Input: part model. Units: mm. Frame: model coordinates. Face numbers are marked on the shaded views. A direction names the side the tool comes from. Round coordinates to 2 decimals unless told otherwise and drop trailing zeros. Loops run counter-clockwise (first coordinate to the right, second up) from the corner with the lowest first, then second, coordinate; pieces in that order, holes last. Notation, with made-up numbers: M 1.5,34.5 L 46.5,34.5 A5 ccw 46.5,42.5 Z; hole C -5,35.5 d7. An arc over 180 degrees is marked long. Use one line per item in the form item = value. Start each with the question number.
Q1. Access query for the marked faces 1 and 2. Directions: +Z, -Z, +X, -X, +Y, -Y. A direction counts if a zero-diameter tool reaches every point of the face in a straight line with its end or side. Return the directions, or none.
Q2. Section query A-A, the plane x = 67.25. Output: boundary loops of the cut face in (y, z), and give its area (3 significant figures).
Q3. Section query B-B, the plane z = -7.75. Output: boundary loops of the cut face in (x, y).
Q4. Ray query, line 1 along Z through (x, y) = (-2, 0); line 2 along Y through (x, z) = (60, -2.15); line 3 along Z through (x, y) = (20, -2). Return the intervals inside material, ascending.
Q5. First-contact query: P1, Ø2, axis at y = -2, z = -15.5, coming from the -X side; P2, Ø10, axis at y = -16.5, z = -7, coming from the +X side; P3, Ø10, axis at x = -7, z = -10.5, coming from the +Y side; P4, Ø18, axis at x = -4.5, y = -9, coming from the -Z side. Flat tips, straight axial feed; report the tip coordinate or a pass-through.
Q6. Mould query, pull axis Z, two halves, no side actions, for the marked faces 3, 4, 5 and 6. Classes: pulls with the +Z half, pulls with the -Z half, needs draft (parallel to the pull), parting line crosses it, or undercut.
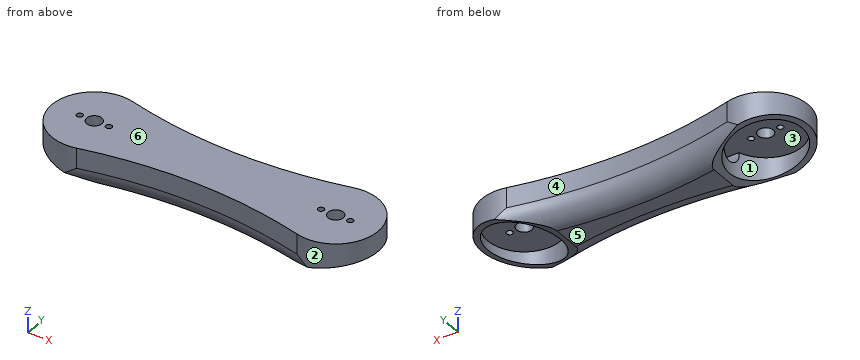
```python
from build123d import *

# Parameters (mm, degrees)
SALIENTE_EXTRUIR1_DEPTH    = 20
CORTAR_EXTRUIR1_DEPTH      = 87.034876649
CORTAR_EXTRUIR1_DEPTH_BACK = 87.034876649
CROQUIS4_R                 = 18
CORTAR_EXTRUIR2_DEPTH      = 14
CROQUIS5_R                 = 3.75
CROQUIS5_R_2               = 1.5
CORTAR_EXTRUIR3_DEPTH      = 85.841027952
REDONDEO1_R                = 10
CORTAR_EXTRUIR4_DEPTH      = 47


with BuildPart() as part:
    # Croquis1 → Saliente-Extruir1 (new body)
    with BuildSketch(Plane.XY):
        with BuildLine():
            ThreePointArc((54.87804878, 20.365795239), (0, 13.570744225), (-54.87804878, 20.365795239))
            ThreePointArc((-54.87804878, 20.365795239), (-81, 0), (-54.87804878, -20.365795239))
            ThreePointArc((-54.87804878, -20.365795239), (0, -13.570744225), (54.87804878, -20.365795239))
            ThreePointArc((54.87804878, -20.365795239), (81, 0), (54.87804878, 20.365795239))
        make_face()
    extrude(amount=-SALIENTE_EXTRUIR1_DEPTH)

    # Croquis2 → Cortar-Extruir1 (cut, two sides: drawn at the far end of the back side and taken through both)
    with BuildSketch(Plane(origin=(0, 0, 0), x_dir=(1, 0, 0), z_dir=(0, 1, 0)).offset(-CORTAR_EXTRUIR1_DEPTH_BACK)):
        with BuildLine():
            Line((-81, 10), (-81, 20))
            Line((-81, 20), (-39, 20))
            ThreePointArc((-39, 20), (-59.790503904, 14.120116398), (-81, 10))
        make_face()
        with BuildLine():
            Line((81, 10), (81, 20))
            Line((81, 20), (39, 20))
            ThreePointArc((39, 20), (59.790503904, 14.120116398), (81, 10))
        make_face()
    extrude(amount=CORTAR_EXTRUIR1_DEPTH + CORTAR_EXTRUIR1_DEPTH_BACK, mode=Mode.SUBTRACT)

    # Croquis4 → Cortar-Extruir2 (cut)
    with BuildSketch(Plane(origin=(0, 0, -20), x_dir=(-1, 0, 0), z_dir=(0, 0, -1))):
        with Locations((60, 0)):
            Circle(CROQUIS4_R)
        with Locations((-60, 0)):
            Circle(CROQUIS4_R)
    extrude(amount=-CORTAR_EXTRUIR2_DEPTH, mode=Mode.SUBTRACT)

    # Croquis5 → Cortar-Extruir3 (cut, through all)
    with BuildSketch(Plane(origin=(0, 0, -6), x_dir=(-1, 0, 0), z_dir=(0, 0, -1))):
        with Locations((60, 0)):
            Circle(CROQUIS5_R)
        with Locations((67.25, 0)):
            Circle(CROQUIS5_R_2)
        with Locations(Location((52.75, 0, 0), (0, 0, 180))):
            Circle(CROQUIS5_R_2)
        with Locations(Location((-67.25, 0, 0), (0, 0, 180))):
            Circle(CROQUIS5_R_2)
        with Locations(Location((-60, 0, 0), (0, 0, 180))):
            Circle(CROQUIS5_R)
        with Locations((-52.75, 0)):
            Circle(CROQUIS5_R_2)
    extrude(amount=-CORTAR_EXTRUIR3_DEPTH, mode=Mode.SUBTRACT)

    # Redondeo1
    # the kernel refuses this fillet: 10 mm, written as the material it takes off along each edge
    with BuildSketch(Plane(origin=(0, -238.570744225, -20), x_dir=(-0.28147080374244887, 0.9595697924802447, 0), z_dir=(-0.9595697924802447, -0.28147080374244887, 0))) as redondeo1_piece_1:
        with BuildLine():
            CenterArc((225 + REDONDEO1_R, -REDONDEO1_R), REDONDEO1_R, 90, 90)
            Line((225, -REDONDEO1_R), (225, 0))
            Line((225, 0), (225 + REDONDEO1_R, 0))
        make_face()
    revolve(axis=Axis((0, -238.570744225, -20), (0, 0, -1)), revolution_arc=32.696012994, mode=Mode.SUBTRACT)
    with BuildSketch(Plane(origin=(0, 238.570744225, -20), x_dir=(0.28147080374244876, -0.9595697924802447, 0), z_dir=(0.9595697924802447, 0.28147080374244876, 0))) as redondeo1_piece_2:
        with BuildLine():
            CenterArc((225 + REDONDEO1_R, -REDONDEO1_R), REDONDEO1_R, 90, 90)
            Line((225 + REDONDEO1_R, 0), (225, 0))
            Line((225, 0), (225, -REDONDEO1_R))
        make_face()
    revolve(axis=Axis((0, 238.570744225, -20), (0, 0, -1)), revolution_arc=32.696012994, mode=Mode.SUBTRACT)

    # Croquis6 → Cortar-Extruir4 (cut, symmetric)
    with BuildSketch(Plane(origin=(0, 0, 0), x_dir=(0, 0, -1), z_dir=(1, 0, 0))):
        with BuildLine():
            Line((6, 5.5), (6, -5.5))
            ThreePointArc((6, -5.5), (13, 0), (6, 5.5))
        make_face()
    extrude(amount=CORTAR_EXTRUIR4_DEPTH, both=True, mode=Mode.SUBTRACT)


solid = part.part
```
Results found:
q1.face_1 = -Z
q1.face_2 = +Z, -Z
q2.outline = M -19.71,-12.46 L -16.48,-12.46 L -16.48,-6 L -1.5,-6 L -1.5,0 L -19.71,0 Z; M 1.5,-6 L 16.48,-6 L 16.48,-12.46 L 19.71,-12.46 L 19.71,0 L 1.5,0 Z
q2.area = 260 mm²
q3.outline = M -54.88,-20.37 A225 cw 54.88,-20.37 A21 ccw long 54.88,20.37 A225 cw -54.88,20.37 A21 ccw long Z; hole M -42.91,-5.65 L 42.91,-5.65 A18 ccw long 42.91,5.65 L -42.91,5.65 A18 ccw long Z
q4.line_1 = -20 to -13, -6 to 0
q4.line_2 = -21 to -3.75, 3.75 to 21
q4.line_3 = -20 to -12.63, -6 to 0
q5.P1 = -42.25
q5.P2 = 77.57
q5.P3 = 13.89
q5.P4 = -20
q6.face_3 = undercut
q6.face_4 = needs draft
q6.face_5 = pulls with the -Z half
q6.face_6 = pulls with the +Z half
